Source: CAD feature listing. Evaluate the final solid. Frame: model axes, mm. Face numbers are marked on the shaded views. Round coordinates to 2 decimals unless told otherwise and drop trailing zeros. Order: outer loops, then holes, each group sorted by start corner. A loop starts at its lowest first (then second) coordinate and runs counter-clockwise, first axis right, second up. Notation, with made-up numbers: (-9, 49) -> (-1, 49) arc R22 ccw to (-1, 87) -> close; hole circle Ø2 at (66.25, 9.25). An arc over 180 degrees is marked (long way). One line per item, written item: value. Start each with the question number.
1) Section C-C (z = 3). Return the cut outline in (x, y) (3 decimals).
2) Ray query, L1, parallel to Y at x = -9.5, z = 2.25; L2, parallel to Z at x = 4.75, y = 8; L3, parallel to X at y = 3, z = 2.35 (3 decimals). Return the intervals inside material, ascending.
3) Section D-D (y = -6.5). Return the cut outline in (x, z) (3 decimals), and give its area (3 significant figures).
4) Mould query, pull axis X, two halves, no side actions, for the marked faces 1, 2 and 3. Classes: pulls with the +X half, pulls with the -X half, needs draft (parallel to the pull), parting line crosses it, or undercut.
5) Pin query (flat end, axial travel): P1, Ø2, axis at y = 0.5, z = 3, coming from the -X side (3 decimals); P2, Ø2.5, axis at x = 9.17, y = -2.65, coming from the +Z side; P3, Ø1, axis at x = -4.5, z = 3, coming from the -Y side. Return the tip coordinate at first contact, or that it passes through.
6) Section B-B (z = 0.95). State how many separate pieces and enclosed holes the cut face has, and give its area (3 significant figures).
7) Section A-A (y = 4.85). Return the cut outline in (x, z) (3 decimals), and give its area (3 significant figures).
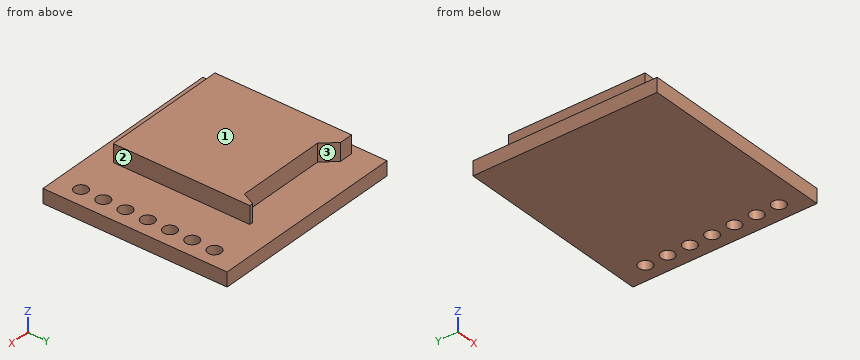
```python
from build123d import *

# Parameters (mm, degrees)
F0_W     = 22.25
F0_H     = 20.7
F1_DEPTH = 1.6
F3_DEPTH = 2
F4_R     = 0.75
F5_DEPTH = 25


with BuildPart() as f1:
    # F0 (on Top) → F1 (new body)
    with BuildSketch(Plane.XY):
        Rectangle(F0_W, F0_H)
    extrude(amount=F1_DEPTH)

    # F2 (on face) → F3 (join)
    with BuildSketch(Plane.XY.offset(1.6)):
        Polygon((-8.493273, 7.25), (-10.025, 7.25), (-10.025, 5.75), (-10.025, -8.1), (4.125, -8.1), (4.125, 5.75), (4.125, 7.25), (3.738537, 7.25), (3.01568, 5.75), (-7.154986, 5.75), align=None)
    extrude(amount=F3_DEPTH)

    # F4 (on face) → F5 (cut)
    with BuildSketch(Plane.XY.offset(1.6)):
        with Locations((9.17196, 7.35)):
            Circle(F4_R)
        with Locations((9.170717, 4.85)):
            Circle(F4_R)
        with Locations((9.169475, 2.350001)):
            Circle(F4_R)
        with Locations((9.168232, -0.149999)):
            Circle(F4_R)
        with Locations((9.16699, -2.649999)):
            Circle(F4_R)
        with Locations((9.165747, -5.149998)):
            Circle(F4_R)
        with Locations((9.164505, -7.649998)):
            Circle(F4_R)
    extrude(amount=-F5_DEPTH, mode=Mode.SUBTRACT)


solid = f1.part
```
Findings:
1. outline: (-10.025, -8.1) -> (4.125, -8.1) -> (4.125, 7.25) -> (3.739, 7.25) -> (3.016, 5.75) -> (-7.155, 5.75) -> (-8.493, 7.25) -> (-10.025, 7.25) -> close
2. L1: -8.1 to 7.25
2. L2: 0 to 1.6
2. L3: -10.025 to 4.125
3. outline: (-11.125, 0) -> (11.125, 0) -> (11.125, 1.6) -> (4.125, 1.6) -> (4.125, 3.6) -> (-10.025, 3.6) -> (-10.025, 1.6) -> (-11.125, 1.6) -> close
3. area: 63.9 mm2
4. face 1: needs draft
4. face 2: pulls with the +X half
4. face 3: undercut
5. P1: x = -10.025
5. P2: z = 1.6
5. P3: y = -8.1
6. separate pieces: 1
6. enclosed holes: 7
6. area: 448 mm2
7. outline: (-11.125, 0) -> (8.421, 0) -> (8.421, 1.6) -> (4.125, 1.6) -> (4.125, 3.6) -> (-10.025, 3.6) -> (-10.025, 1.6) -> (-11.125, 1.6) -> close; (9.921, 0) -> (11.125, 0) -> (11.125, 1.6) -> (9.921, 1.6) -> close
7. area: 61.5 mm2
